Drawing for the job (mm, zero at the part's lowest x, y, z). Coordinates: 2 decimals unless noted, no trailing zeros. Order: outer loops, then holes, each group sorted by start corner. A loop starts at its lowest first (then second) coordinate and runs counter-clockwise, first axis right, second up. Notation, with made-up numbers: (26.25, -8) -> (68.25, -8) arc R24 cw to (68.25, 18) -> close; hole circle Ø3 at (14.25, 11.5). An arc over 180 degrees is marked (long way). Write each question's results on one line, items separated by ' | '.
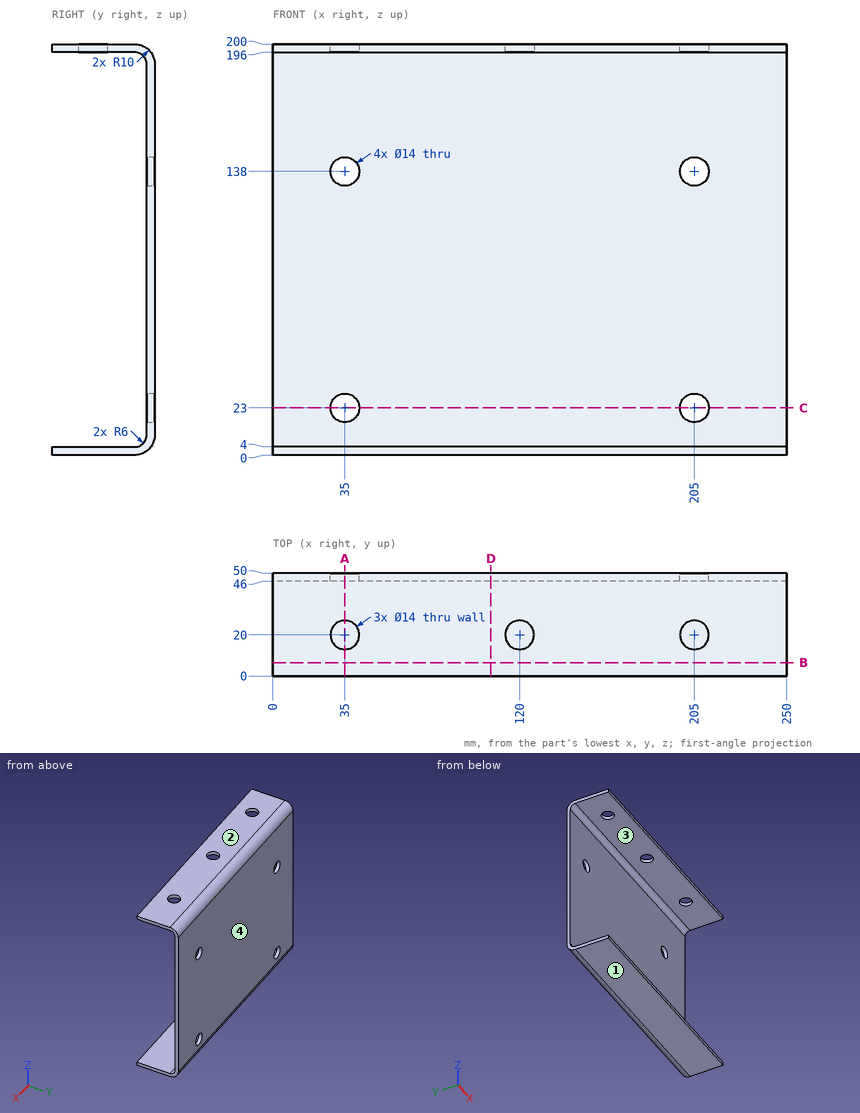
Item 1: Slice it at D-D, the plane x = 106. List the corners of the cut face in (y, z).
Answer:
outline: (0, 0) -> (40, 0) arc R10 ccw to (50, 10) -> (50, 190) arc R10 ccw to (40, 200) -> (0, 200) -> (0, 196) -> (40, 196) arc R6 cw to (46, 190) -> (46, 10) arc R6 cw to (40, 4) -> (0, 4) -> close
Item 2: Slice it at C-C, the plane z = 23. List the corners of the cut face in (x, y), and give its area (3 significant figures).
Answer:
outline: (0, 46) -> (28, 46) -> (28, 50) -> (0, 50) -> close; (42, 46) -> (198, 46) -> (198, 50) -> (42, 50) -> close; (212, 46) -> (250, 46) -> (250, 50) -> (212, 50) -> close | area: 888 mm^2
Item 3: Slice it at B-B, the plane y = 6.5. List the corners of the cut face in (x, z), and give its area (3 significant figures).
Answer:
outline: (0, 0) -> (250, 0) -> (250, 4) -> (0, 4) -> close; (0, 196) -> (250, 196) -> (250, 200) -> (0, 200) -> close | area: 2,000 mm^2
Item 4: Drill centre lines: line 1 (X direction, y = 49.15, z = 23); line 2 (Z direction, x = 160.5, y = 39); line 3 (Y direction, x = 175, z = 32). Where is each one in solid material? Low to high. Write a range as from..to.
Answer:
line 1: x = 0..28, 42..198, 212..250 | line 2: z = 0..4, 196..200 | line 3: y = 46..50
Item 5: Pin check, flat tips, straight feed: pin 1 (8 mm diameter, centred on x = 163, z = 138, fed in from -Y); pin 2 (11 mm diameter, centred on x = 35, y = 20, fed in from +Z). Stop position of each tip, or through.
Answer:
pin 1: stops at y = 46 | pin 2: stops at z = 4
Item 6: Slice it at A-A, the plane x = 35. List the corners of the cut face in (y, z).
Answer:
outline: (0, 0) -> (40, 0) arc R10 ccw to (50, 10) -> (50, 16) -> (46, 16) -> (46, 10) arc R6 cw to (40, 4) -> (0, 4) -> close; (0, 196) -> (13, 196) -> (13, 200) -> (0, 200) -> close; (27, 196) -> (40, 196) arc R6 cw to (46, 190) -> (46, 145) -> (50, 145) -> (50, 190) arc R10 ccw to (40, 200) -> (27, 200) -> close; (46, 30) -> (50, 30) -> (50, 131) -> (46, 131) -> close
Item 7: Pull direction Z, two halves, no side cores. Call the marked faces 1, 2, 3 and 4: released by +Z, released by -Z, zero draft, split by the parting line, or undercut.
Answer:
face 1: released by -Z | face 2: released by +Z | face 3: undercut | face 4: zero draft
